Autodesk Inventor part; units mm, degrees
ref_plane "YZ Plane" through (0, 0, 0) normal (1, 0, 0) x (0, 1, 0)
ref_plane "XZ Plane" through (0, 0, 0) normal (0, 1, 0) x (-1, 0, 0)
ref_plane "XY Plane" through (0, 0, 0) normal (0, 0, 1) x (1, 0, 0)
sketch "Sketch1" plane through (0, 0, 0) normal (0, 1, 0) x (-1, 0, 0)
  line L0 (0, 0) -> (3, 0)
  line L1 (3, 0) -> (3, -106)
  line L2 (3, -106) -> (0, -106)
  line L3 (0, -106) -> (0, 0)
  line L4 (0, -53) -> (-80, -53) construction
  line L5 (-80, -51.5) -> (0, -51.5)
  line L6 (0, -51.5) -> (0, -54.5)
  line L7 (0, -54.5) -> (-80, -54.5)
  line L8 (-80, -54.5) -> (-80, -51.5)
  line L9 (-80, -51.5) -> (0, -54.5) construction
  line L10 (0, -51.5) -> (-80, -54.5) construction
  point P0 (-40, -53)
  dimension "d0" = 3
  dimension "d1" = 106
  dimension "d2" = 80
  dimension "d3" = 3
extrude "Extrusion1" add sketch "Sketch1" along normal blind 70
sketch "Sketch2" plane through (-3, 0, -106) normal (-1, 0, 0) x (0, 0, 1)
  line L0 (0, 0) -> (106, 0)
  line L1 (0, 70) -> (106, 70)
  line L2 (106, 0) -> (103, 0)
  line L3 (103, 0) -> (103, 70)
  line L4 (103, 70) -> (106, 70)
  line L5 (106, 70) -> (106, 0)
  dimension "d6" = 3
sketch "Sketch3" plane through (-3, 0, -106) normal (-1, 0, 0) x (0, 0, 1)
  line L0 (51.5, 70) -> (0, 70)
  line L1 (0, 0) -> (3, 0)
  line L2 (3, 0) -> (3, 70)
  line L3 (3, 70) -> (0, 70)
  line L4 (0, 70) -> (0, 0)
  point P0 (106, 0)
  dimension "d7" = 3
sketch "Sketch4" plane through (-3, 0, -106) normal (-1, 0, 0) x (0, 0, 1)
  line L0 (51.5, 0) -> (0, 0)
  line L1 (51.5, 70) -> (0, 70)
  line L2 (0, 0) -> (3, 0)
  line L3 (3, 0) -> (3, 70)
  line L4 (3, 70) -> (0, 70)
  line L5 (0, 70) -> (0, 0)
  point P0 (106, 0)
  dimension "d8" = 3
extrude "Extrusion2" add sketch "Sketch2" along normal blind 4
extrude "Extrusion3" add sketch "Sketch4" along normal blind 4
sketch "Sketch5" plane through (-3, 0, -3) normal (-1, 0, 0) x (0, 0, 1)
  line L0 (-103, 0) -> (-103, 70) construction
  line L1 (-103, 70) -> (3, 70) construction
  line L2 (3, 70) -> (-50, 70) construction
  line L3 (-50, 70) -> (-50, 82.7) construction
  circle A0 centre (-50, 82.7) radius 12.7
  circle A1 centre (-50, 82.7) radius 17.5
  point P0 (3, 0)
  dimension "d13" = 12.7
  dimension "d14" = 25.4
  dimension "d15" = 35
extrude "Extrusion4" add sketch "Sketch5" against normal blind 20
sketch "Sketch6" plane through (80, 0, -51.5) normal (1, 0, 0) x (0, 0, -1)
  circle A0 centre (1.5, 82.7) radius 12.7
  circle A1 centre (1.5, 82.7) radius 12.7
  circle A2 centre (1.5, 82.7) radius 17.5
  point P0 (-51.5, 0)
  point P1 (1.5, 70)
extrude "Extrusion5" add sketch "Sketch6" against normal blind 20
sketch "Sketch7" plane through (80, 0, -51.5) normal (1, 0, 0) x (0, 0, -1)
  arc A0 (3, 65.2644) -> (0, 65.2644) centre (1.5, 82.7) ccw
  line L0 (1.5, 82.7) -> (-23.0448, 82.7)
  line L1 (-23.0448, 82.7) -> (-23.0448, 99.7436)
  line L2 (-23.0448, 99.7436) -> (1.5, 99.7436)
  line L3 (1.5, 99.7436) -> (1.5, 82.7)
  line L4 (-23.0448, 82.7) -> (23.5266, 82.7)
  line L5 (23.5266, 82.7) -> (23.5266, 103.3181)
  line L6 (23.5266, 103.3181) -> (-23.0448, 103.3181)
  line L7 (-23.0448, 103.3181) -> (-23.0448, 82.7)
  point P0 (-51.5, 0)
extrude "Extrusion6" cut sketch "Sketch7" against normal blind 2000
sketch "Sketch8" plane through (80, 82.7, -65.7) normal (0, 1, 0) x (1, 0, 0)
  line L0 (-83, -25.4) -> (-83, 0)
  line L1 (-83, 0) -> (-63, 0)
  line L2 (-63, 0) -> (-63, 15)
  line L3 (-63, 15) -> (-83, 15)
  line L4 (-83, 15) -> (-83, 0)
  line L5 (0, 0) -> (-20, 0)
  line L6 (0, 0) -> (-20, 0)
  line L7 (-20, 0) -> (-20, 15)
  line L8 (-20, 15) -> (0, 15)
  line L9 (0, 15) -> (0, 0)
  line L10 (-20, -25.4) -> (0, -25.4)
  line L11 (-20, -25.4) -> (0, -25.4)
  line L12 (0, -25.4) -> (0, -40.4)
  line L13 (0, -40.4) -> (-20, -40.4)
  line L14 (-20, -40.4) -> (-20, -25.4)
  line L15 (-83, -25.4) -> (-63, -25.4)
  line L16 (-63, -25.4) -> (-63, -40.4)
  line L17 (-63, -40.4) -> (-83, -40.4)
  line L18 (-83, -40.4) -> (-83, -25.4)
  point P0 (-80, -65.7)
  dimension "d22" = 15
  dimension "d23" = 15
  dimension "d24" = 15
  dimension "d25" = 20
extrude "Extrusion7" add sketch "Sketch8" against normal blind 5
fillet "Fillet1" radius 2 12 edges at (0, 32.6322, -54.5) (0, 66.7372, -60.1721) (8.5, 65.2644, -54.5) (17, 67.6322, -54.5) (70, 65.2644, -54.5) (60, 67.6322, -54.5) (0, 32.6322, -51.5) (8.5, 65.2644, -51.5) (0, 66.7372, -45.8279) (17, 67.6322, -51.5) (70, 65.2644, -51.5) (60, 67.6322, -51.5)
sketch "Sketch9" plane through (0, 70, 0) normal (0, 1, 0) x (1, 0, 0)
  arc A0 (17.0325, 56.141) -> (19, 54.5) centre (19, 56.5) ccw
  line L0 (60, 49.5) -> (60, 53)
  line L1 (17.0325, 56.141) -> (60, 56.141)
  line L2 (60, 56.141) -> (60, 49.5)
  line L3 (60, 49.5) -> (17.0325, 49.5)
  line L4 (17.0325, 49.5) -> (17.0325, 56.141)
  point P0 (0, 0)
extrude "Extrusion8" cut sketch "Sketch9" against normal blind 7.5
sketch "Sketch10" plane through (-3, 82.7, -40.3) normal (0, 1, 0) x (1, 0, 0)
  line L0 (20, -4.0705) -> (20, -15)
  line L1 (0, 0) -> (20, 0)
  line L2 (20, -15) -> (0, -15)
  line L3 (0, -15) -> (0, 0)
  line L4 (0, 0) -> (20, 0)
  line L5 (20, 0) -> (20, -15)
  line L6 (20, -15) -> (0, -15) construction
  line L7 (10, -15) -> (10, 40.4) construction
  line L8 (0, 40.4) -> (20, 40.4) construction
  line L9 (0, -15) -> (10, 0) construction
  line L10 (0, 0) -> (10, -15) construction
  line L11 (20, 0) -> (10, -15) construction
  line L12 (20, -15) -> (10, 0) construction
  line L13 (20, 25.4) -> (0, 25.4) construction
  line L14 (10, 25.4) -> (0, 40.4) construction
  line L15 (0, 62.7) -> (0, -37.3) construction
  line L16 (0, 25.4) -> (10, 40.4) construction
  line L17 (10, 40.4) -> (20, 25.4) construction
  line L18 (20, 25.4) -> (15, 32.9) construction
  line L19 (20, 40.4) -> (20, 25.4) construction
  line L20 (10, 25.4) -> (20, 40.4) construction
  circle A0 centre (5, -7.5) radius 3.175
  circle A1 centre (15, -7.5) radius 3.175
  circle A2 centre (5, 32.9) radius 3.175
  circle A3 centre (15, 32.9) radius 3.175
  point P0 (3, -40.3)
  dimension "d31" = 6.35
  dimension "d32" = 6.35
  dimension "d33" = 6.35
  dimension "d34" = 6.35
extrude "Extrusion9" cut sketch "Sketch10" against normal blind 7.5 contours A0 | A1 | A2 | A3
sketch "Sketch11" plane through (60, 82.7, -40.3) normal (0, 1, 0) x (1, 0, 0)
  line L0 (20, -15) -> (0, -15) construction
  line L1 (10, -15) -> (10, 40.4) construction
  line L2 (0, 40.4) -> (20, 40.4) construction
  line L3 (0, 40.4) -> (10, 25.4) construction
  line L4 (20, 25.4) -> (0, 25.4) construction
  line L5 (5, 32.9) -> (20, 32.9) construction
  line L6 (20, 40.4) -> (20, 29.4705) construction
  line L7 (10, 25.4) -> (20, 40.4) construction
  line L8 (0, -15) -> (10, 0) construction
  line L9 (0, 0) -> (20, 0) construction
  line L10 (0, 0) -> (10, -15) construction
  line L11 (20, 0) -> (20, -15) construction
  line L12 (10, -15) -> (20, 0) construction
  line L13 (20, 0) -> (10, 0) construction
  line L14 (20, -15) -> (10, 0) construction
  circle A0 centre (5, -7.5) radius 3.175
  circle A1 centre (15, -7.5) radius 3.175
  circle A2 centre (5, 32.9) radius 3.175
  circle A3 centre (15, 32.9) radius 3.175
  point P0 (-60, -40.3)
  dimension "d37" = 6.35
  dimension "d38" = 6.35
  dimension "d39" = 6.35
  dimension "d40" = 6.35
extrude "Extrusion10" cut sketch "Sketch11" against normal blind 7.5
properties part number "scopeHolderv2"
Geometry: final body of the model. Coordinates: model frame, mm. A direction names the side the tool comes from. Round coordinates to 2 decimals unless told otherwise and drop trailing zeros. Order: outer loops, then holes, each group sorted by start corner. A loop starts at its lowest first (then second) coordinate and runs counter-clockwise, first axis right, second up. Notation, with made-up numbers: M 38,48.5 L 97,48.5 A11 ccw 97,69.5 Z; hole C 49,83 d8. An arc over 180 degrees is marked long. Use one line per item in the form item = value. Start each with the question number.
Q1. Mould query, pull axis X, two halves, no side actions, for faces 6 (the face through (70, 77.7, -77)), 7 (the face through (-7, 35, -2)), 8 (the face through (1.59, 80.24, -76.35)), 9 (the face through (0, 35, -25)). Classes: +X half, -X half, draft (parallel to the pull), parting line (faces both ways), or undercut.
Q2. Material intervals for line 1 (X direction, y = 79.2, z = -32.8) (3 decimals); line 2 (Z direction, x = 65, y = 80) (3 decimals); line 3 (Z direction, x = 42, y = 56.5), sorted ascending. Write a range as [from, to].
Q3. Cut plane D-D (x = 70.5). Return loops of the section in (y, z), and give its area (3 significant figures).
Q4. Cut plane B-B (x = 12). Count the separate pieces of the cut face and the enclosed holes in it, and give its area (3 significant figures).
Q5. Cut plane A-A (z = -73.2). Return loops of the section in (x, y) (3 decimals).
Q6. Access query for faces 1 (the face through (-5, 35, -103)), 2 (the face through (17.032, 67, -53)), 3 (the face through (70, 77.7, -30)), 4 (the face through (7, 77.7, -77)), 5 (the face through (70.14, 69.76, -41.22)). Directions: +Z, -Z, +X, -X, +Y, -Y. A direction counts if a zero-diameter tool reaches every point of the face in a straight line with its end or side. Return the directions, or none.
Q7. Cut plane C-C (y = 15.5). Return loops of the section in (x, z), and give its area (3 significant figures).
Q8. Pin query (flat end, axial travel): pin 1 Ø7.5 at (x, z) = (12, -32.8) entering from +Y; pin 2 Ø3 at (x, y) = (20, 48) entering from -Z; pin 3 Ø3.5 at (x, z) = (65.5, -29.5) entering from -Y; pin 4 Ø12 at (y, z) = (58, -72.5) entering from -X. Return the tip coordinate at first contact, or that it passes through.
Geometry results:
q1.face_6 = draft
q1.face_7 = -X half
q1.face_8 = undercut
q1.face_9 = +X half
q2.line_1 = [-3, -1.175], [5.175, 8.825], [15.175, 17], [60, 61.825], [68.175, 71.825], [78.175, 80]
q2.line_2 = [-80.7, -76.375], [-70.025, -65.41], [-40.59, -35.975], [-29.625, -25.3]
q2.line_3 = [-54.5, -51.5]
q3.outline = M 0,-54.5 L 63.52,-54.5 A2 cw 65.48,-56.14 A17.5 ccw 77.7,-69.77 L 77.7,-80.7 L 82.7,-80.7 L 82.7,-65.7 A12.7 cw 82.7,-40.3 L 82.7,-25.3 L 77.7,-25.3 L 77.7,-36.23 A17.5 ccw 65.48,-49.86 A2 cw 63.52,-51.5 L 0,-51.5 Z
q3.area = 529 mm^2
q4.separate_pieces = 3
q4.enclosed_holes = 0
q4.area = 465 mm^2
q5.outline = M -3,0 L 0,0 L 0,70 L -3,70 Z; M -3,77.7 L -1.175,77.7 L -1.175,82.7 L -3,82.7 Z; M 5.175,77.7 L 8.825,77.7 L 8.825,82.7 L 5.175,82.7 Z; M 15.175,77.7 L 17,77.7 L 17,82.7 L 15.175,82.7 Z; M 60,77.7 L 61.825,77.7 L 61.825,82.7 L 60,82.7 Z; M 68.175,77.7 L 71.825,77.7 L 71.825,82.7 L 68.175,82.7 Z; M 78.175,77.7 L 80,77.7 L 80,82.7 L 78.175,82.7 Z
q6.face_1 = -X, +Y, -Y
q6.face_2 = +Z, -Z, +Y
q6.face_3 = +Z, +X, -X, -Y
q6.face_4 = -Z, +X, -X
q6.face_5 = +Z, +X, -Y
q7.outline = M -7,-106 L 0,-106 L 0,-56.5 A2 cw 2,-54.5 L 80,-54.5 L 80,-51.5 L 2,-51.5 A2 cw 0,-49.5 L 0,0 L -7,0 L -7,-3 L -3,-3 L -3,-103 L -7,-103 Z
q7.area = 584 mm^2
q8.pin_1 = 82.7
q8.pin_2 = -54.5
q8.pin_3 = 77.7
q8.pin_4 = -3
